from build123d import *

# Parameters (mm, degrees)
PAD_DEPTH     = 1.75
SKETCH001_W   = 2.85
SKETCH001_H   = 4
PAD001_DEPTH  = 0.5
SKETCH002_W   = 4.33
SKETCH002_H   = 4.97
SKETCH002_W_2 = 4.97
SKETCH002_H_2 = 4.33
PAD002_DEPTH  = 1.5
SKETCH003_W   = 1.57
SKETCH003_H   = 2.26
SKETCH003_W_2 = 2.37
SKETCH003_H_2 = 3.28
SKETCH003_W_3 = 1.48
SKETCH003_H_3 = 3.07
SKETCH003_W_4 = 2.29
SKETCH003_H_4 = 1.09
SKETCH003_W_5 = 2.26
SKETCH003_H_5 = 1.57
SKETCH003_W_6 = 3.07
SKETCH003_H_6 = 1.48
SKETCH003_W_7 = 3.75
SKETCH003_H_7 = 1.73
PAD003_DEPTH  = 0.75


with BuildPart() as part:
    # Sketch → Pad (new body)
    with BuildSketch(Plane.XY):
        with BuildLine():
            Line((-7.75, 22.25), (-7.75, -22.25))
            ThreePointArc((-7.75, -22.25), (-6.944544, -24.194544), (-5, -25))
            Line((-5, -25), (5, -25))
            ThreePointArc((5, -25), (6.944544, -24.194544), (7.75, -22.25))
            Line((7.75, -22.25), (7.75, 22.25))
            ThreePointArc((7.75, 22.25), (6.944544, 24.194544), (5, 25))
            Line((5, 25), (-5, 25))
            ThreePointArc((-5, 25), (-6.944544, 24.194544), (-7.75, 22.25))
        make_face()
    extrude(amount=PAD_DEPTH)

    # Sketch001 (on Face10 of Pad) → Pad001 (join)
    with BuildSketch(Plane.XY.offset(1.75)):
        with Locations((-6.115, 17.21)):
            Rectangle(SKETCH001_W, SKETCH001_H)
        with Locations((-2.755, 22.53)):
            Rectangle(SKETCH001_W, SKETCH001_H)
        with Locations((1.985, 22.53)):
            Rectangle(SKETCH001_W, SKETCH001_H)
        with Locations((6.155, 17.21)):
            Rectangle(SKETCH001_W, SKETCH001_H)
        with Locations((-6.115, -0.19)):
            Rectangle(SKETCH001_W, SKETCH001_H)
        with Locations((-6.115, -18.5)):
            Rectangle(SKETCH001_W, SKETCH001_H)
    extrude(amount=PAD001_DEPTH)

    # Sketch002 (on Face5 of Pad001) → Pad002 (join)
    with BuildSketch(Plane.XY.offset(1.75)):
        with Locations((1.625, 5.325)):
            Rectangle(SKETCH002_W, SKETCH002_H)
        with Locations((-1.375, -10.795)):
            Rectangle(SKETCH002_W_2, SKETCH002_H_2)
        with Locations((4.775, -10.795)):
            Rectangle(SKETCH002_W_2, SKETCH002_H_2)
        with Locations((-1.375, -19.615)):
            Rectangle(SKETCH002_W_2, SKETCH002_H_2)
        with Locations((4.775, -19.615)):
            Rectangle(SKETCH002_W_2, SKETCH002_H_2)
    extrude(amount=PAD002_DEPTH)

    # Sketch003 (on Face5 of Pad002) → Pad003 (join)
    with BuildSketch(Plane.XY.offset(1.75)):
        with Locations((-2.775, -3.885)):
            Rectangle(SKETCH003_W, SKETCH003_H)
        with Locations((-0.605, -3.885)):
            Rectangle(SKETCH003_W_2, SKETCH003_H_2)
        with Locations((2.48, -3.885)):
            Rectangle(SKETCH003_W_3, SKETCH003_H_3)
        with Locations((4.46, -3.885)):
            Rectangle(SKETCH003_W_3, SKETCH003_H_3)
        with Locations((6.44, -3.885)):
            Rectangle(SKETCH003_W_3, SKETCH003_H_3)
        with Locations((-5.685, 5.965)):
            Rectangle(SKETCH003_W_4, SKETCH003_H_4)
        with Locations((-5.685, 8.295)):
            Rectangle(SKETCH003_W_5, SKETCH003_H_5)
        with Locations((-5.685, 3.68)):
            Rectangle(SKETCH003_W_6, SKETCH003_H_6)
        with Locations((-6.62, 11.525)):
            Rectangle(SKETCH003_W_3, SKETCH003_H_3)
        with Locations((-4.64, 11.525)):
            Rectangle(SKETCH003_W_3, SKETCH003_H_3)
        with Locations((-2.66, 11.525)):
            Rectangle(SKETCH003_W_3, SKETCH003_H_3)
        with Locations((-0.68, 11.525)):
            Rectangle(SKETCH003_W_3, SKETCH003_H_3)
        with Locations((1.745, 11.525)):
            Rectangle(SKETCH003_W_2, SKETCH003_H_2)
        with Locations((4.215, 11.525)):
            Rectangle(SKETCH003_W, SKETCH003_H)
        with Locations((6.285, 11.525)):
            Rectangle(SKETCH003_W, SKETCH003_H)
        with Locations((0.245, 0.015)):
            Rectangle(SKETCH003_W_7, SKETCH003_H_7)
    extrude(amount=PAD003_DEPTH)


solid = part.part
For this review, take the finished solid that the model builds, in its own axes (mm). A direction names the side the tool comes from. Coordinates: 2 decimals unless noted, no trailing zeros. Loops run counter-clockwise (first coordinate to the right, second up) from the corner with the lowest first, then second, coordinate; pieces in that order, holes last. Notation, with made-up numbers: (-21, 39.5) - (1, 39.5) arc R32 cw to (1, 76.5) - close; hole circle Ø8 at (49, 77.5). An arc over 180 degrees is marked (long way). Use a Markdown table: item, result. Add a question column.
Item 1: We need section D-D (y = 16). Give the boundary of the cut face in (x, z), and give its area (3 significant figures).
Item 2: We need section C-C (y = -4). Give the boundary of the cut face in (x, z).
Item 3: For line 1 (Y direction, x = -3.25, z = 2.2) (3 decimals); line 2 (X direction, y = 21.5, z = 1.8); line 3 (Z direction, x = -6, y = 22), list the stretches that pass through material, from the lowest coordinate up.
Item 4: We need section B-B (y = -20). Give the boundary of the cut face in (x, z).
Item 5: Tool access review of faces 4 (the face through (-6, 6, 2.5)), 5 (the face through (-6, 0, 2.25)), 6 (the face through (-3, 23, 2.25)), 7 (the face through (5, -8.63, 2)): name each direction out of +Z, -Z, +X, -X, +Y, -Y from which nothing blocks a thin tool from reaching the whole face with its end or side.
Item 6: We need section A-A (y = 5). Give the boundary of the cut face in (x, z), and give its area (3 significant figures).
Item 7: Mouldability with a two-part tool opening along X and no side actions: class faces 1 (the face through (7.26, -20, 2)), 2 (the face through (4, 12, 2.5)), 3 (the face through (1.11, -11, 2)) as pulls with the +X half, pulls with the -X half, needs draft (parallel to the pull), parting line crosses it, or undercut.
Item 8: Insertion check: pin 1 Ø1.2 at (x, y) = (-5, 4) entering from +Z; pin 2 Ø1.2 at (y, z) = (-20, 2.5) entering from -X. Each pin has a flat end and moves straight along its axis. Give the tip position at first contact, or say it passes through.
Results list:
| question | item | result |
|---|---|---|
| 1 | outline | (-7.75, 0) - (7.75, 0) - (7.75, 1.75) - (7.58, 1.75) - (7.58, 2.25) - (4.73, 2.25) - (4.73, 1.75) - (-4.69, 1.75) - (-4.69, 2.25) - (-7.54, 2.25) - (-7.54, 1.75) - (-7.75, 1.75) - close |
| 1 | area | 30.0 mm^2 |
| 2 | outline | (-7.75, 0) - (7.75, 0) - (7.75, 1.75) - (7.18, 1.75) - (7.18, 2.5) - (5.7, 2.5) - (5.7, 1.75) - (5.2, 1.75) - (5.2, 2.5) - (3.72, 2.5) - (3.72, 1.75) - (3.22, 1.75) - (3.22, 2.5) - (1.74, 2.5) - (1.74, 1.75) - (0.58, 1.75) - (0.58, 2.5) - (-1.79, 2.5) - (-1.79, 1.75) - (-1.99, 1.75) - (-1.99, 2.5) - (-3.56, 2.5) - (-3.56, 1.75) - (-7.75, 1.75) - close |
| 3 | line 1 | y = -21.78 to -17.45, -12.96 to -8.63, -5.015 to -2.755, 9.99 to 13.06, 20.53 to 24.53 |
| 3 | line 2 | x = -4.18 to -1.33, 0.56 to 3.41 |
| 3 | line 3 | z = 0 to 1.75 |
| 4 | outline | (-7.75, 0) - (7.75, 0) - (7.75, 1.75) - (7.26, 1.75) - (7.26, 3.25) - (2.29, 3.25) - (2.29, 1.75) - (1.11, 1.75) - (1.11, 3.25) - (-3.86, 3.25) - (-3.86, 1.75) - (-4.69, 1.75) - (-4.69, 2.25) - (-7.54, 2.25) - (-7.54, 1.75) - (-7.75, 1.75) - close |
| 5 | face 4 | +Z, -X, +Y, -Y |
| 5 | face 5 | +Z, -X, -Y |
| 5 | face 6 | +Z, +X, -X, +Y |
| 5 | face 7 | +Z, +X, -X |
| 6 | outline | (-7.75, 0) - (7.75, 0) - (7.75, 1.75) - (3.79, 1.75) - (3.79, 3.25) - (-0.54, 3.25) - (-0.54, 1.75) - (-7.75, 1.75) - close |
| 6 | area | 33.6 mm^2 |
| 7 | face 1 | pulls with the +X half |
| 7 | face 2 | needs draft |
| 7 | face 3 | undercut |
| 8 | pin 1 | stops at z = 2.5 |
| 8 | pin 2 | stops at x = -7.54 |
